```python
from build123d import *

# Parameters (mm, degrees)
SKETCH1_R           = 30
SKETCH1_R_2         = 15
BOSS_EXTRUDE1_DEPTH = 36
SKETCH2_W           = 94.945060367
SKETCH2_H           = 33
BOSS_EXTRUDE2_DEPTH = 16.5
CUT_EXTRUDE1_DEPTH  = 45
FILLET1_R           = 7
SKETCH4_R           = 15
BOSS_EXTRUDE3_DEPTH = 22.5


with BuildPart() as part:
    # Sketch1 → Boss-Extrude1 (new body)
    with BuildSketch(Plane(origin=(0, 0, 0), x_dir=(1, 0, 0), z_dir=(0, 1, 0))):
        Circle(SKETCH1_R)
        Circle(SKETCH1_R_2, mode=Mode.SUBTRACT)
    extrude(amount=-BOSS_EXTRUDE1_DEPTH)

    # Sketch2 → Boss-Extrude2 (add, symmetric)
    with BuildSketch(Plane(origin=(0, -18, 0), x_dir=(1, 0, 0), z_dir=(0, 1, 0))):
        with Locations((72.527469817, 0)):
            Rectangle(SKETCH2_W, SKETCH2_H)
    extrude(amount=BOSS_EXTRUDE2_DEPTH, both=True)

    # Sketch3 → Cut-Extrude1 (cut)
    with BuildSketch(Plane(origin=(120, 0, 0), x_dir=(0, 0, -1), z_dir=(1, 0, 0))):
        Polygon((5.5, -1.5), (16.5, -12.5), (16.5, -1.5), align=None)
        Polygon((16.5, -34.5), (16.5, -23.5), (5.5, -34.5), align=None)
        Polygon((-16.5, -34.5), (-5.5, -34.5), (-16.5, -23.5), align=None)
        Polygon((-16.5, -1.5), (-16.5, -12.5), (-5.5, -1.5), align=None)
    extrude(amount=-CUT_EXTRUDE1_DEPTH, mode=Mode.SUBTRACT)

    # Fillet1
    fillet1_edges = [part.edges().sort_by_distance(p)[0] for p in [
        (75, -7, 11),
        (75, -29, 11),
        (75, -29, -11),
        (75, -7, -11),
    ]]
    fillet(fillet1_edges, radius=FILLET1_R)

    # Sketch4 → Boss-Extrude3 (add, symmetric)
    with BuildSketch(Plane(origin=(120, 0, 0), x_dir=(0, 0, -1), z_dir=(1, 0, 0))):
        with Locations((0, -18)):
            Circle(SKETCH4_R)
    extrude(amount=BOSS_EXTRUDE3_DEPTH, both=True)


solid = part.part
```
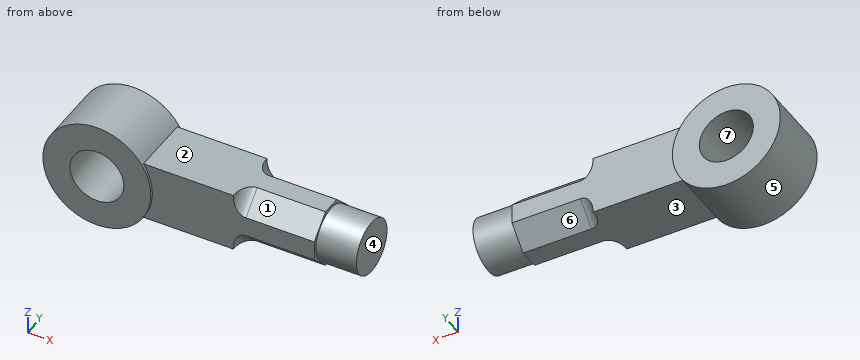
Build history of the part. All positions in model axes, mm. Face numbers are marked on the shaded views. A direction names the side the tool comes from. Give positions to 0.01 mm unless a question says otherwise; leave off trailing zeros. Loops run counter-clockwise (first coordinate to the right, second up) from the corner with the lowest first, then second, coordinate; pieces in that order, holes last. Notation, with made-up numbers: (-24.5, 83) -> (-13.5, 83) arc R27 cw to (-13.5, 99) -> close; hole circle Ø11 at (-38, -7). An arc over 180 degrees is marked (long way). One line per question, with ' | ' between items.
Q1. Drill centre lines: line 1 along Z through (x, y) = (0, -20); line 2 along X through (y, z) = (-14, 0); line 3 along X through (y, z) = (-2.5, 0.5). Where is each one in solid material? Low to high. Write a range as [from, to].
Filled sheet:
line 1: z = [-30, -15], [15, 30] | line 2: x = [-30, -15], [15, 142.5] | line 3: x = [-30, -14.99], [14.99, 120]
Q2. Drop flat-ended pins along their axis: pin 1 (5 mm diameter, centred on y = -32.5, z = 15.5, fed in from -X); pin 2 (2 mm diameter, centred on y = -5.5, z = -20, fed in from +X); pin 3 (0.6 mm diameter, centred on y = -34, z = -16, fed in from +X); pin 4 (18 mm diameter, centred on x = 0, z = 0, fed in from +Y). Give the stop position or say it passes through.
Filled sheet:
pin 1: stops at x = -27.04 | pin 2: stops at x = 23.22 | pin 3: stops at x = 75 | pin 4: passes through
Q3. Cut at D-D, the plane x = 96.5. Write the cut outline in (y, z).
Filled sheet:
outline: (-34.5, -5.5) -> (-23.5, -16.5) -> (-12.5, -16.5) -> (-1.5, -5.5) -> (-1.5, 5.5) -> (-12.5, 16.5) -> (-23.5, 16.5) -> (-34.5, 5.5) -> close
Q4. Cut at B-B, the plane x = -11. Write the cut outline in (y, z).
Filled sheet:
outline: (-36, -27.91) -> (0, -27.91) -> (0, -10.2) -> (-36, -10.2) -> close; (-36, 10.2) -> (0, 10.2) -> (0, 27.91) -> (-36, 27.91) -> close
Q5. Cut at C-C, the plane y = -18. Write the cut outline in (x, z).
Filled sheet:
outline: (25.05, -16.5) -> (120, -16.5) -> (120, -15) -> (142.5, -15) -> (142.5, 15) -> (120, 15) -> (120, 16.5) -> (25.05, 16.5) arc R30 ccw (long way) to start; hole circle Ø30 at (0, 0)
Q6. Tool access for the marked faces 1, 2 and 3: list every direction of +Z, -Z, +X, -X, +Y, -Y with a clear straight run to the whole face (end or side of a thin tool).
Filled sheet:
face 1: +Z, +X, -Y | face 2: +Z, +X, +Y, -Y | face 3: -Z, +X, +Y, -Y
Q7. Pull direction X, two halves, no side cores. Call the marked faces 4, 5, 6 and 7: pulls with the +X half, pulls with the -X half, needs draft (parallel to the pull), parting line crosses it, or undercut.
Filled sheet:
face 4: pulls with the +X half | face 5: parting line crosses it | face 6: needs draft | face 7: undercut
Q8. Cut at A-A, the plane z = 0. Write the cut outline in (x, y), plus the area to 4 significant figures.
Filled sheet:
outline: (-30, -36) -> (-15, -36) -> (-15, 0) -> (-30, 0) -> close; (15, -36) -> (30, -36) -> (30, -34.5) -> (120, -34.5) -> (120, -33) -> (142.5, -33) -> (142.5, -3) -> (120, -3) -> (120, -1.5) -> (30, -1.5) -> (30, 0) -> (15, 0) -> close | area: 4,725 mm²
